Drawing for the job (mm, zero at the part's lowest x, y, z). A direction names the side the tool comes from. Give positions to 0.01 mm unless a question says otherwise; leave off trailing zeros. Order: outer loops, then holes, each group sorted by start corner. A loop starts at its lowest first (then second) coordinate and runs counter-clockwise, first axis right, second up. Notation, with made-up numbers: (65.25, -32.5) - (120.25, -32.5) arc R18 cw to (120.25, 0.5) - close; hole circle Ø6 at (39.5, 56.5). An arc over 180 degrees is marked (long way). One line per item, written item: value.
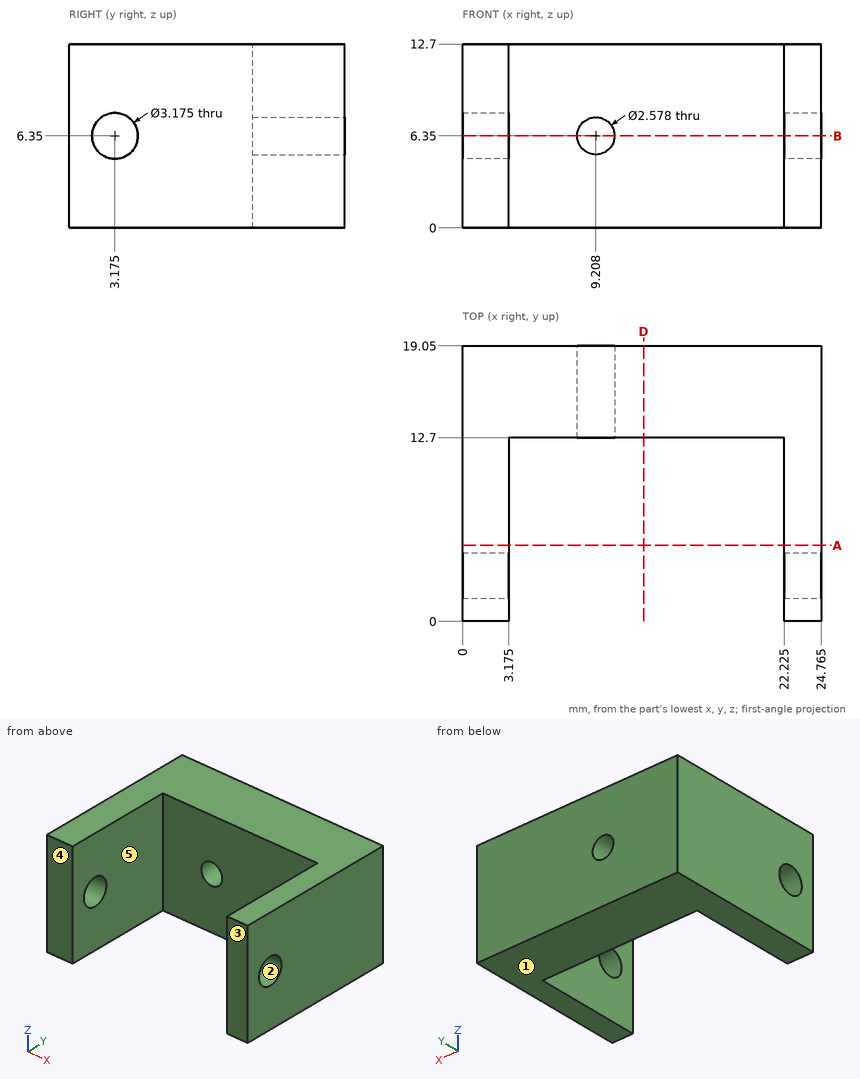
(1) Slice it at B-B, the plane z = 6.35. Count the separate pieces of the cut face and the enclosed holes in it, and give its area (3 significant figures).
Completed:
separate pieces: 4
enclosed holes: 0
area: 195 mm²
(2) Drill centre lines: line 1 (X direction, y = 6.25, z = 11.25) (1 decimal); line 2 (Y direction, x = 23, z = 6.35); line 3 (X direction, y = 14, z = 6.35) (1 decimal). Where is each one in solid material? Low to high.
Completed:
line 1: 0 to 3.2, 22.2 to 24.8
line 2: 0 to 1.59, 4.76 to 19.05
line 3: 0 to 7.9, 10.5 to 24.8
(3) Slice it at D-D, the plane x = 12.5. Give the cut face in (y, z).
Completed:
outline: (12.7, 0) - (19.05, 0) - (19.05, 12.7) - (12.7, 12.7) - close
(4) Pin check, flat tip, straight feed: P1, Ø6, axis at x = 7.5, y = 7, coming from the -Z side. Stop position of the tip, or through.
Completed:
P1: through
(5) 3-axis set-ups, long thin cutter, end or side, ignore diameter. For the marked faces 4 and 5: which of +Z, -Z, +X, -X, +Y, -Y reach the whole face in a straight line?
Completed:
face 4: +Z, -Z, +X, -X, -Y
face 5: +Z, -Z, -Y
(6) Slice it at A-A, the plane y = 5.25. Give the cut face in (x, z) (1 decimal).
Completed:
outline: (0, 0) - (3.2, 0) - (3.2, 12.7) - (0, 12.7) - close; (22.2, 0) - (24.8, 0) - (24.8, 12.7) - (22.2, 12.7) - close
(7) Pull direction Z, two halves, no side cores. Call the marked faces 1, 2 and 3: +Z half, -Z half, draft (parallel to the pull), parting line (faces both ways), or undercut.
Completed:
face 1: -Z half
face 2: undercut
face 3: draft
